Geometry check sheet. Reference: the model listing, model coordinates, mm. A direction names the side the tool comes from. Round coordinates to 2 decimals unless told otherwise and drop trailing zeros. Order: outer loops, then holes, each group sorted by start corner. A loop starts at its lowest first (then second) coordinate and runs counter-clockwise, first axis right, second up.
(1) Set-up check for faces 1 (the face through (6.186, 2.902, 18.868)), 2 (the face through (20, 0, 50)), 3 (the face through (37.5, 4, 80)), 4 (the face through (3, 4, 20)): record each of +Z, -Z, +X, -X, +Y, -Y from which the full face is reachable in a straight line by a thin tool's end or side.
(2) Cross-section at B-B on z = 25. Enter the section's corners in (x, y).
(3) Gauge pin test, flat ends, axial feed: P1, Ø0.5, axis at x = 38.5, y = 4, coming from the +Z side; P2, Ø0.5, axis at x = 39.5, y = 4, coming from the -Z side; P3, Ø8, axis at x = 30.5, y = 5, coming from the +Z side. Record the tip position at first contact, or that the pin passes through.
(4) Cross-section at A-A on x = 27.5. Enter the section's corners in (y, z), and give its area (3 significant figures).
(5) Cross-section at C-C on y = 7.5. Enter the section's corners in (x, z), and give its area (3 significant figures).
(6) Thickness scan on L1, parallel to X at y = 3.25, z = 51; L2, parallel to Z at x = 21.5, y = 7; L3, parallel to Z at x = 25, y = 0.5. Record the ranges inside material, lowest first.
(7) Draft check along Z on faces 5 (the face through (19.967, -3.547, 15.313)), 6 (the face through (19.967, -3.547, 84.687)), 7 (the face through (39, 0, 50)), 8 (the face through (3, 4, 80)). Enter one of: pulls with the +Z half, pulls with the -Z half, needs draft (parallel to the pull), parting line crosses it, or undercut.
(8) Cross-section at D-D on x = 8. Enter the section's corners in (y, z).
from build123d import *

# Parameters (mm, degrees)
PAD_DEPTH       = 40.5
POCKET_DEPTH    = 14.001
CHAMFER_SIZE    = 2
POCKET001_DEPTH = 3
POCKET002_DEPTH = 3
POCKET003_DEPTH = 40.501
CHAMFER001_SIZE = 1


with BuildPart() as part:
    # Sketch → Pad (new body)
    with BuildSketch(Plane.YZ):
        Polygon((10, 9), (10, 91), (-4, 85), (-4, 15), align=None)
    extrude(amount=PAD_DEPTH)

    # Sketch001 (on Face1 of Pad) → Pocket (cut, through all)
    with BuildSketch(Plane(origin=(0, -4, 0), x_dir=(0, 0, -1), z_dir=(0, -1, 0))):
        Polygon((-78.838843, 37.5), (-21.161157, 37.5), (-50, 21.954061), align=None)
        Polygon((-82, 35.795939), (-53.161157, 20.25), (-82, 4.704061), align=None)
        Polygon((-21.161157, 3), (-78.838843, 3), (-50, 18.545939), align=None)
        Polygon((-46.838843, 20.25), (-18, 35.795939), (-18, 4.704061), align=None)
    extrude(amount=-POCKET_DEPTH, mode=Mode.SUBTRACT)

    # Chamfer
    chamfer_edges = [part.edges().sort_by_distance(p)[0] for p in [
        (3, 3, 78.838843),
        (18.545939, 3, 50),
        (35.795939, 3, 18),
        (20.25, 3, 46.838843),
        (37.5, 3, 78.838843),
        (4.704061, 3, 18),
        (37.5, 3, 21.161157),
        (21.954061, 3, 50),
        (4.704061, 3, 82),
        (20.25, 3, 53.161157),
        (35.795939, 3, 82),
        (3, 3, 21.161157),
    ]]
    chamfer(chamfer_edges, length=CHAMFER_SIZE)

    # Sketch002 (on Face10 of Chamfer) → Pocket001 (cut)
    with BuildSketch(Plane.YZ.offset(40.5)):
        Polygon((3.693853, 80.739104), (3.260896, 80.306147), (3.260896, 79.693853), (3.693853, 79.260896), (4.306147, 79.260896), (4.739104, 79.693853), (4.739104, 80.306147), (4.306147, 80.739104), align=None)
        Polygon((3.693853, 50.739104), (3.260896, 50.306147), (3.260896, 49.693853), (3.693853, 49.260896), (4.306147, 49.260896), (4.739104, 49.693853), (4.739104, 50.306147), (4.306147, 50.739104), align=None)
        Polygon((3.693853, 20.739104), (3.260896, 20.306147), (3.260896, 19.693853), (3.693853, 19.260896), (4.306147, 19.260896), (4.739104, 19.693853), (4.739104, 20.306147), (4.306147, 20.739104), align=None)
        Polygon((-1.693853, 69.260896), (-1.260896, 69.693853), (-1.260896, 70.306147), (-1.693853, 70.739104), (-2.306147, 70.739104), (-2.739104, 70.306147), (-2.739104, 69.693853), (-2.306147, 69.260896), align=None)
        Polygon((-1.693853, 29.260896), (-1.260896, 29.693853), (-1.260896, 30.306147), (-1.693853, 30.739104), (-2.306147, 30.739104), (-2.739104, 30.306147), (-2.739104, 29.693853), (-2.306147, 29.260896), align=None)
    extrude(amount=-POCKET001_DEPTH, mode=Mode.SUBTRACT)

    # Sketch003 (on Face9 of Pocket001) → Pocket002 (cut)
    with BuildSketch(Plane.YZ):
        Polygon((3.693853, 80.739104), (3.260896, 80.306147), (3.260896, 79.693853), (3.693853, 79.260896), (4.306147, 79.260896), (4.739104, 79.693853), (4.739104, 80.306147), (4.306147, 80.739104), align=None)
        Polygon((3.693853, 50.739104), (3.260896, 50.306147), (3.260896, 49.693853), (3.693853, 49.260896), (4.306147, 49.260896), (4.739104, 49.693853), (4.739104, 50.306147), (4.306147, 50.739104), align=None)
        Polygon((3.693853, 20.739104), (3.260896, 20.306147), (3.260896, 19.693853), (3.693853, 19.260896), (4.306147, 19.260896), (4.739104, 19.693853), (4.739104, 20.306147), (4.306147, 20.739104), align=None)
        Polygon((-1.693853, 69.260896), (-1.260896, 69.693853), (-1.260896, 70.306147), (-1.693853, 70.739104), (-2.306147, 70.739104), (-2.739104, 70.306147), (-2.739104, 69.693853), (-2.306147, 69.260896), align=None)
        Polygon((-1.693853, 29.260896), (-1.260896, 29.693853), (-1.260896, 30.306147), (-1.693853, 30.739104), (-2.306147, 30.739104), (-2.739104, 30.306147), (-2.739104, 29.693853), (-2.306147, 29.260896), align=None)
    extrude(amount=POCKET002_DEPTH, mode=Mode.SUBTRACT)

    # Sketch004 → Pocket003 (cut, through all)
    with BuildSketch(Plane(origin=(0, 0, 0), x_dir=(0, 1, 0), z_dir=(-1, 0, 0))):
        Polygon((-4, -32), (0, -36), (0, -64), (-4, -68), align=None)
    extrude(amount=-POCKET003_DEPTH, mode=Mode.SUBTRACT)

    # Chamfer001
    chamfer001_edges = [part.edges().sort_by_distance(p)[0] for p in [
        (20.25, 10, 91),
        (20.25, 10, 9),
        (0, 10, 50),
        (40.5, 10, 50),
        (20.25, -4, 85),
        (20.25, -4, 15),
    ]]
    chamfer(chamfer001_edges, length=CHAMFER001_SIZE)


solid = part.part
Found:
1. face 1: +Y, -Y
1. face 2: +X, -X, -Y
1. face 3: +X
1. face 4: -X
2. outline: (0, -4) - (3, -4) - (3, 10) - (1, 10) - (0, 9) - close; (5.07, -4) - (8.48, -4) - (8.48, 10) - (5.07, 10) - close; (32.02, -4) - (35.43, -4) - (35.43, 10) - (32.02, 10) - close; (37.5, -4) - (40.5, -4) - (40.5, 9) - (39.5, 10) - (37.5, 10) - close
3. P1: stops at z = 88.54
3. P2: stops at z = 11.46
3. P3: stops at z = 90.57
4. outline: (-4, 16) - (-3.08, 14.61) - (9.08, 9.39) - (10, 10) - (10, 18) - (-4, 18) - close; (-4, 82) - (10, 82) - (10, 90) - (9.08, 90.61) - (-3.08, 85.39) - (-4, 84) - close; (-2.61, 33.39) - (10, 33.39) - (10, 39.71) - (0, 39.71) - (0, 36) - close; (-2.61, 66.61) - (0, 64) - (0, 60.29) - (10, 60.29) - (10, 66.61) - close
4. area: 299 mm2
5. outline: (0, 10.07) - (40.5, 10.07) - (40.5, 89.93) - (0, 89.93) - close; hole (3, 23.16) - (3.95, 22.92) - (17.6, 48.24) - (17.6, 51.76) - (3.95, 77.08) - (3, 76.84) - close; hole (5.65, 19.76) - (6.7, 18) - (33.8, 18) - (34.85, 19.76) - (21.2, 45.08) - (19.3, 45.08) - close; hole (5.65, 80.24) - (19.3, 54.92) - (21.2, 54.92) - (34.85, 80.24) - (33.8, 82) - (6.7, 82) - close; hole (22.9, 48.24) - (36.55, 22.92) - (37.5, 23.16) - (37.5, 76.84) - (36.55, 77.08) - (22.9, 51.76) - close
5. area: 1,460 mm2
6. L1: x = 0 to 3, 17.6 to 22.9, 37.5 to 40.5
6. L2: z = 10.29 to 18, 44.52 to 55.48, 82 to 89.71
6. L3: z = 13.07 to 18, 38.03 to 44.35, 55.65 to 61.97, 82 to 86.93
7. face 5: pulls with the -Z half
7. face 6: pulls with the +Z half
7. face 7: undercut
7. face 8: undercut
8. outline: (-4, 16) - (-3.08, 14.61) - (9.08, 9.39) - (10, 10) - (10, 18) - (-4, 18) - close; (-4, 24.11) - (10, 24.11) - (10, 30.44) - (-4, 30.44) - close; (-4, 69.56) - (10, 69.56) - (10, 75.89) - (-4, 75.89) - close; (-4, 82) - (10, 82) - (10, 90) - (9.08, 90.61) - (-3.08, 85.39) - (-4, 84) - close
